from build123d import *

# Parameters (mm, degrees)
SKETCH1_W                                     = 38.5
SKETCH1_H                                     = 140
BASE_FLANGE1_DEPTH                            = 4.93522
EDGE_FLANGE1_STRIP_W                          = 29.90088
EDGE_FLANGE1_STRIP_H                          = 4.93522
EDGE_FLANGE1_STRIP_CUT_DEPTH                  = 140
EDGE_FLANGE1_DEPTH                            = 140
EDGE_FLANGE2_STRIP_W                          = 29.90088
EDGE_FLANGE2_STRIP_H                          = 4.93522
EDGE_FLANGE2_STRIP_CUT_DEPTH                  = 84
EDGE_FLANGE2_RELIEF_W                         = 32.36849
EDGE_FLANGE2_RELIEF_H                         = 2.46761
EDGE_FLANGE2_RELIEF_CUT_DEPTH                 = 4.93522
EDGE_FLANGE2_DEPTH                            = 84
FILLET1_R                                     = 12
CUT_EXTRUDE1_REACH                            = 92.308
SKETCH20_W                                    = 25.53239
SKETCH20_H                                    = 8
FILLET2_R                                     = 5
FILLET1_OF_MIRROR1_R                          = 12
FILLET2_OF_MIRROR1_R                          = 5
CSK_FOR_M10_FLAT_HEAD_MACHINE_SCREW1_AT_COUNT = 2
CSK_FOR_M10_FLAT_HEAD_MACHINE_SCREW1_AT_PITCH = 52.021630117
CSK_FOR_M10_FLAT_HEAD_MACHINE_SCREW1_2_COUNT  = 2
CSK_FOR_M10_FLAT_HEAD_MACHINE_SCREW1_2_PITCH  = 104.043260233
CSK_FOR_M10_FLAT_HEAD_MACHINE_SCREW1_3_COUNT  = 2
CSK_FOR_M10_FLAT_HEAD_MACHINE_SCREW1_3_PITCH  = 85
CSK_FOR_M10_FLAT_HEAD_MACHINE_SCREW1_4_COUNT  = 2
CSK_FOR_M10_FLAT_HEAD_MACHINE_SCREW1_4_PITCH  = 60


# Sheet-metal steps are written as plain solids
with BuildPart() as part:
    # Sketch1 → Base-Flange1 (new body)
    with BuildSketch(Plane(origin=(0, 0, 0), x_dir=(1, 0, 0), z_dir=(0, 1, 0))):
        Rectangle(SKETCH1_W, SKETCH1_H)
    extrude(amount=-BASE_FLANGE1_DEPTH)

    # Edge-Flange1 strip (across the edge) → Edge-Flange1 strip cut (cut)
    with BuildSketch(Plane(origin=(-19.25, 0, -70), x_dir=(1, 0, 0), z_dir=(0, 0, 1))):
        with Locations((-9.87044, -2.46761)):
            Rectangle(EDGE_FLANGE1_STRIP_W, EDGE_FLANGE1_STRIP_H)
    edge_flange1_strip_cut = extrude(amount=EDGE_FLANGE1_STRIP_CUT_DEPTH, mode=Mode.SUBTRACT)

    # Edge-Flange1 section (across the edge) → Edge-Flange1 (add)
    with BuildSketch(Plane(origin=(-19.25, 0, -70), x_dir=(1, 0, 0), z_dir=(0, 0, 1))):
        with BuildLine():
            Line((-4.93522, 5.08), (-4.93522, 37))
            Line((-4.93522, 37), (0, 37))
            Line((0, 37), (0, 5.08))
            ThreePointArc((0, 5.08), (1.487897552, 1.487897552), (5.08, 0))
            Line((5.08, 0), (5.08, -4.93522))
            ThreePointArc((5.08, -4.93522), (-2.001829977, -2.001829977), (-4.93522, 5.08))
        make_face()
    edge_flange1 = extrude(amount=EDGE_FLANGE1_DEPTH)

    # Edge-Flange2 strip (across the edge) → Edge-Flange2 strip cut (cut)
    with BuildSketch(Plane(origin=(-24.18522, 37, 42), x_dir=(0, -1, 0), z_dir=(0, 0, -1))):
        with Locations((-4.93522, -2.46761)):
            Rectangle(EDGE_FLANGE2_STRIP_W, EDGE_FLANGE2_STRIP_H)
    edge_flange2_strip_cut = extrude(amount=EDGE_FLANGE2_STRIP_CUT_DEPTH, mode=Mode.SUBTRACT)

    # Edge-Flange2 relief (on the sheet) → Edge-Flange2 relief cut (cut)
    with BuildSketch(Plane(origin=(-24.18522, 26.98478, 42), x_dir=(0, -1, 0), z_dir=(-1, 0, 0))):
        with Locations((-13.716635, 1.233805)):
            Rectangle(EDGE_FLANGE2_RELIEF_W, EDGE_FLANGE2_RELIEF_H)
        with Locations((-13.716635, -85.233805)):
            Rectangle(EDGE_FLANGE2_RELIEF_W, EDGE_FLANGE2_RELIEF_H)
    edge_flange2_relief_cut = extrude(amount=-EDGE_FLANGE2_RELIEF_CUT_DEPTH, mode=Mode.SUBTRACT)

    # Edge-Flange2 section (across the edge) → Edge-Flange2 (add)
    with BuildSketch(Plane(origin=(-24.18522, 37, 42), x_dir=(0, -1, 0), z_dir=(0, 0, -1))):
        with BuildLine():
            Line((0, 5.08), (0, 30.31478))
            Line((0, 30.31478), (4.93522, 30.31478))
            Line((4.93522, 30.31478), (4.93522, 5.08))
            ThreePointArc((4.93522, 5.08), (6.423117552, 1.487897552), (10.01522, 0))
            Line((10.01522, 0), (10.01522, -4.93522))
            ThreePointArc((10.01522, -4.93522), (2.933390023, -2.001829977), (0, 5.08))
        make_face()
    edge_flange2 = extrude(amount=EDGE_FLANGE2_DEPTH)

    # Fillet1
    fillet1_edges = [part.edges().sort_by_distance(p)[0] for p in [
        (-54.5, 34.53239, 42),
        (-54.5, 34.53239, -42),
    ]]
    fillet(fillet1_edges, radius=FILLET1_R)

    # Sketch20 → Cut-Extrude1 (cut, up to next)
    with BuildSketch(Plane.ZY.offset(24.18522), mode=Mode.PRIVATE) as cut_extrude1_sk1:
        with Locations((-57.233805, 33)):
            Rectangle(SKETCH20_W, SKETCH20_H)
    cut_extrude1_tool1 = extrude(cut_extrude1_sk1.sketch, amount=-CUT_EXTRUDE1_REACH, mode=Mode.PRIVATE) & part.part
    # Sketch20 → Cut-Extrude1 (cut, up to next)
    with BuildSketch(Plane.ZY.offset(24.18522), mode=Mode.PRIVATE) as cut_extrude1_sk2:
        with Locations((57.233805, 33)):
            Rectangle(SKETCH20_W, SKETCH20_H)
    cut_extrude1_tool2 = extrude(cut_extrude1_sk2.sketch, amount=-CUT_EXTRUDE1_REACH, mode=Mode.PRIVATE) & part.part
    cut_extrude1_1 = cut_extrude1_tool1.solids().sort_by_distance((-24.18522, 33, -57.233805))[0]
    add(cut_extrude1_1, mode=Mode.SUBTRACT)
    cut_extrude1_2 = cut_extrude1_tool2.solids().sort_by_distance((-24.18522, 33, 57.233805))[0]
    add(cut_extrude1_2, mode=Mode.SUBTRACT)
    cut_extrude1 = cut_extrude1_1 + cut_extrude1_2  # Cut-Extrude1 as one shape, for the pattern or mirror that repeats it

    # Fillet2
    fillet2_edges = [part.edges().sort_by_distance(p)[0] for p in [
        (-21.71761, 29, -70),
        (-21.71761, 29, 70),
    ]]
    fillet(fillet2_edges, radius=FILLET2_R)

    # Mirror1: Edge-Flange1 strip cut, Edge-Flange1, Edge-Flange2 strip cut, Edge-Flange2 relief cut, Edge-Flange2, Cut-Extrude1 across plane
    add(edge_flange1_strip_cut.mirror(Plane(origin=(0, 0, 0), x_dir=(0, 0, 1), z_dir=(1, 0, 0))), mode=Mode.SUBTRACT)
    add(edge_flange1.mirror(Plane(origin=(0, 0, 0), x_dir=(0, 0, 1), z_dir=(1, 0, 0))))
    add(edge_flange2_strip_cut.mirror(Plane(origin=(0, 0, 0), x_dir=(0, 0, 1), z_dir=(1, 0, 0))), mode=Mode.SUBTRACT)
    add(edge_flange2_relief_cut.mirror(Plane(origin=(0, 0, 0), x_dir=(0, 0, 1), z_dir=(1, 0, 0))), mode=Mode.SUBTRACT)
    add(edge_flange2.mirror(Plane(origin=(0, 0, 0), x_dir=(0, 0, 1), z_dir=(1, 0, 0))))
    add(cut_extrude1.mirror(Plane(origin=(0, 0, 0), x_dir=(0, 0, 1), z_dir=(1, 0, 0))), mode=Mode.SUBTRACT)

    # Fillet1 of Mirror1
    fillet1_of_mirror1_edges = [part.edges().sort_by_distance(p)[0] for p in [
        (54.5, 34.53239, 42),
        (54.5, 34.53239, -42),
    ]]
    fillet(fillet1_of_mirror1_edges, radius=FILLET1_OF_MIRROR1_R)

    # Fillet2 of Mirror1
    fillet2_of_mirror1_edges = [part.edges().sort_by_distance(p)[0] for p in [
        (21.71761, 29, -70),
        (21.71761, 29, 70),
    ]]
    fillet(fillet2_of_mirror1_edges, radius=FILLET2_OF_MIRROR1_R)

    # Sketch30 → CSK for M10 Flat Head Machine Screw1 (revolve, cut)
    with BuildSketch(Plane(origin=(42.5, 32.06478, 30), x_dir=(0, 0, -1), z_dir=(1, 0, 0))):
        Polygon((0, 0), (0, 4.93522), (5.5, 4.93522), (5.5, 4.5), (10, 0), align=None)
    csk_for_m10_flat_head_machine_screw1 = revolve(axis=Axis((42.5, 25.71478, 30), (0, 1, 0)), mode=Mode.SUBTRACT)

    # CSK for M10 Flat Head Machine Screw1 at: CSK for M10 Flat Head Machine Screw1 ×2
    with Locations(*[Vector(-0.8169678632647617, 0, -0.5766831975986554) * (i * CSK_FOR_M10_FLAT_HEAD_MACHINE_SCREW1_AT_PITCH) for i in range(1, CSK_FOR_M10_FLAT_HEAD_MACHINE_SCREW1_AT_COUNT)]):
        add(csk_for_m10_flat_head_machine_screw1, mode=Mode.SUBTRACT)

    # CSK for M10 Flat Head Machine Screw1 2: CSK for M10 Flat Head Machine Screw1 ×2
    with Locations(*[Vector(-0.8169678632647617, 0, -0.5766831975986554) * (i * CSK_FOR_M10_FLAT_HEAD_MACHINE_SCREW1_2_PITCH) for i in range(1, CSK_FOR_M10_FLAT_HEAD_MACHINE_SCREW1_2_COUNT)]):
        add(csk_for_m10_flat_head_machine_screw1, mode=Mode.SUBTRACT)

    # CSK for M10 Flat Head Machine Screw1 3: CSK for M10 Flat Head Machine Screw1 ×2
    with Locations(*[(-i * CSK_FOR_M10_FLAT_HEAD_MACHINE_SCREW1_3_PITCH, 0, 0) for i in range(1, CSK_FOR_M10_FLAT_HEAD_MACHINE_SCREW1_3_COUNT)]):
        add(csk_for_m10_flat_head_machine_screw1, mode=Mode.SUBTRACT)

    # CSK for M10 Flat Head Machine Screw1 4: CSK for M10 Flat Head Machine Screw1 ×2
    with Locations(*[(0, 0, -i * CSK_FOR_M10_FLAT_HEAD_MACHINE_SCREW1_4_PITCH) for i in range(1, CSK_FOR_M10_FLAT_HEAD_MACHINE_SCREW1_4_COUNT)]):
        add(csk_for_m10_flat_head_machine_screw1, mode=Mode.SUBTRACT)


solid = part.part
Design review of the part built by this model. Coordinates are the model's own, in mm. A direction names the side the tool comes from. Give positions to 0.01 mm unless a question says otherwise; leave off trailing zeros. Loops run counter-clockwise (first coordinate to the right, second up) from the corner with the lowest first, then second, coordinate; pieces in that order, holes last. Notation, with made-up numbers: M 43,43.25 L 58,43.25 A26 cw 58,79.25 Z; hole C 55,-37.5 d6. An arc over 180 degrees is marked long. Answer as a JSON object with one key per item and string values.
Item 1: Mouldability with a two-part tool opening along X and no side actions: class faces 4 (the face through (46.02, 36.28, 34.59)), 5 (the face through (-22, 27, 44.468)), 6 (the face through (24.185, 17, -1)) as pulls with the +X half, pulls with the -X half, needs draft (parallel to the pull), parting line crosses it, or undercut.
Output values:
{"face 4": "undercut", "face 5": "needs draft", "face 6": "pulls with the +X half"}
Item 2: We need section B-B (z = -8). State the section outline as (x, y) points.
Output values:
{"outline": "M -54.5,32.06 L -29.27,32.06 A5.08 cw -24.19,26.98 L -24.19,5.08 A10.02 ccw -14.17,-4.94 L 14.17,-4.94 A10.02 ccw 24.19,5.08 L 24.19,26.98 A5.08 cw 29.27,32.06 L 54.5,32.06 L 54.5,37 L 29.27,37 A10.02 ccw 19.25,26.98 L 19.25,5.08 A5.08 cw 14.17,0 L -14.17,0 A5.08 cw -19.25,5.08 L -19.25,26.98 A10.02 ccw -29.27,37 L -54.5,37 Z"}
Item 3: We need section C-C (x = 21.5). State the section outline as (y, z) points, and give its area (3 significant figures).
Output values:
{"outline": "M -1.74,-70 L 24,-70 A5 ccw 29,-65 L 29,-44.47 L 24.52,-44.47 L 24.52,-42 L 33.31,-42 L 33.31,42 L 24.52,42 L 24.52,44.47 L 29,44.47 L 29,65 A5 ccw 24,70 L -1.74,70 Z", "area": "4,630 mm2"}
Item 4: Machinability: for faces 1 (the face through (0, 0, -1)), 2 (the face through (22, 29, 55)), 3 (the face through (-22, 29, -55)), which of the approach directions +Z, -Z, +X, -X, +Y, -Y give a long, thin tool a straight path to every point of the face, cutting with its end or side? Answer none if there is none.
Output values:
{"face 1": "+Z, -Z, +Y", "face 2": "+Z, +X, -X, +Y", "face 3": "-Z, +X, -X, +Y"}
Item 5: Wall thickness on line 1 along X through (y, z) = (16, 34); line 2 along X through (y, z) = (27.5, 27); line 3 along Z through (x, y) = (-42, 36): over which ranges is each line inside the solid? List them lowest first.
Output values:
{"line 1": "x = -24.19 to -19.25, 19.25 to 24.19", "line 2": "x = -24.21 to -19.26, 19.26 to 24.21", "line 3": "z = -42 to -36.04, -23.96 to 23.96, 36.04 to 42"}
Item 6: For P1, Ø19, axis at y = 18.5, z = -0.5, coming from the -X side; P2, Ø10, axis at x = -9.5, z = -44.5, coming from the +Y side; P3, Ø5, axis at y = 24.5, z = 34, coming from the +X side; P4, Ø5, axis at x = -21, y = 26, coming from the -Z side, all flat-tipped, find the tip position at first contact; note any pin that passes through.
Output values:
{"P1": "stops at x = -24.29", "P2": "stops at y = 0.01", "P3": "stops at x = 24.19", "P4": "stops at z = -70"}
Item 7: We need section A-A (y = 7.5). State the section outline as (x, z) points, and give its area (3 significant figures).
Output values:
{"outline": "M -24.19,-70 L -19.25,-70 L -19.25,70 L -24.19,70 Z; M 19.25,-70 L 24.19,-70 L 24.19,70 L 19.25,70 Z", "area": "1,380 mm2"}
